Design review of the part built by this model. Coordinates are the model's own, in mm. Face numbers are marked on the shaded views. A direction names the side the tool comes from. Coordinates: 2 decimals unless noted, no trailing zeros. Order: outer loops, then holes, each group sorted by start corner. A loop starts at its lowest first (then second) coordinate and runs counter-clockwise, first axis right, second up. Notation, with made-up numbers: M 35,-15.5 L 56,-15.5 A29 ccw 56,14.5 Z; hole C 48,64.25 d9. An arc over 180 degrees is marked long. Answer as a JSON object with one key per item and string values.
from build123d import *

# Parameters (mm, degrees)
F1_DEPTH    = 25.4
F2_T1_DEPTH = 50.8
F3_R        = 5.08


# Not quite as in the source:
# - a fillet or chamfer that OpenCascade refuses, or shapes differently, is made with other operations: its cross-section is extruded or revolved along the edge and cut away or added


with BuildPart() as f1:
    # F0 (on Front) → F1 (new body)
    with BuildSketch(Plane.XZ):
        Polygon((0, 31.75), (0, 0), (50.8, 0), (50.8, 6.35), (6.35, 6.35), (6.35, 31.75), align=None)
    extrude(amount=-F1_DEPTH)

    # F2: fillet of radius 5.08 on 2 edges, made by hand

    # F2_s2 → F2_t1 (cut)
    with BuildSketch(Plane.XZ.offset(-38.1)):
        with BuildLine():
            ThreePointArc((50.8, 1.27), (49.3121024484, 4.8621024484), (45.72, 6.35))
            Line((45.72, 6.35), (50.8, 6.35))
            Line((50.8, 6.35), (50.8, 1.27))
        make_face()
        with BuildLine():
            ThreePointArc((45.72, 0), (49.3121024484, 1.4878975516), (50.8, 5.08))
            Line((50.8, 5.08), (50.8, 0))
            Line((50.8, 0), (45.72, 0))
        make_face()
    extrude(amount=F2_T1_DEPTH, mode=Mode.SUBTRACT)

    # F3
    f3_edges = [f1.edges().sort_by_distance(p)[0] for p in [
        (0, 12.7, 31.75),
    ]]
    fillet(f3_edges, radius=F3_R)


solid = f1.part
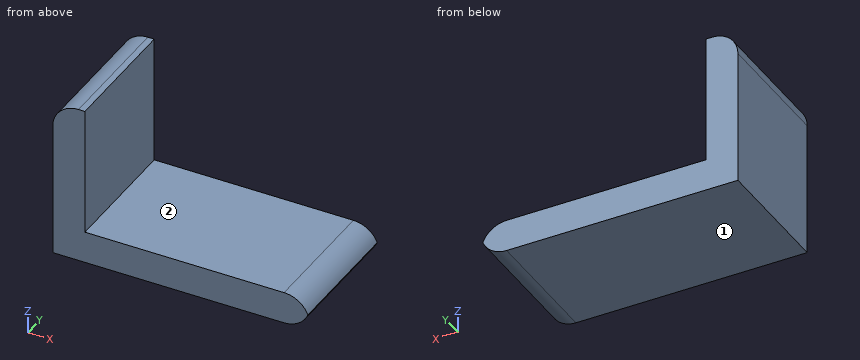
1) Tool access review of the marked faces 1 and 2: name each direction out of +Z, -Z, +X, -X, +Y, -Y from which nothing blocks a thin tool from reaching the whole face with its end or side.
Taken from the geometry:
{"face 1": "-Z, +X, -X, +Y, -Y", "face 2": "+Z, +X, +Y, -Y"}
2) Insertion check: pin 1 Ø7.5 at (y, z) = (17.5, 17) entering from +X; pin 2 Ø12.5 at (x, y) = (28.5, 18.5) entering from +Z; pin 3 Ø8 at (x, z) = (33, 13.5) entering from -Y; pin 4 Ø5 at (y, z) = (19.5, 6) entering from +X. Each pin has a flat end and moves straight along its axis. Give the tip position at first contact, or say it passes through.
Taken from the geometry:
{"pin 1": "stops at x = 6.35", "pin 2": "stops at z = 6.35", "pin 3": "passes through", "pin 4": "stops at x = 50.28"}
3) To check wall thickness, follow L1, parallel to X at y = 4, z = 18; L2, parallel to X at y = 15.5, z = 2.5. State the ranges of each line that lie inside material, in increasing order.
Taken from the geometry:
{"L1": "x = 0 to 6.35", "L2": "x = 0 to 50.1"}
4) Add section C-C (x = 28). State the section outline as (y, z) points, and give its area (3 significant figures).
Taken from the geometry:
{"outline": "M 0,0 L 25.4,0 L 25.4,6.35 L 0,6.35 Z", "area": "161 mm2"}
5) Add section A-A (y = 3.25). State the section outline as (x, z) points (3 decimals), and give its area (3 significant figures).
Taken from the geometry:
{"outline": "M 0,0 L 45.72,0 A5.08 ccw 50.429,3.175 A5.08 ccw 45.72,6.35 L 6.35,6.35 L 6.35,31.75 L 5.08,31.75 A5.08 ccw 0,26.67 Z", "area": "468 mm2"}
6) Add section B-B (z = 16). State the section outline as (x, y) points, and give its area (3 significant figures).
Taken from the geometry:
{"outline": "M 0,0 L 6.35,0 L 6.35,25.4 L 0,25.4 Z", "area": "161 mm2"}
